```python
from build123d import *

# Parameters (mm, degrees)
SKETCH1_R             = 4.05
BOSS_EXTRUDE1_DEPTH   = 10
SKETCH2_W             = 18
SKETCH2_H             = 10
BOSS_EXTRUDE2_DEPTH   = 25
F_4_CLEARANCE_HOLE1_D = 3.2639


with BuildPart() as part:
    # Sketch1 → Boss-Extrude1 (new, symmetric)
    with BuildSketch(Plane.XY):
        with BuildLine():
            Line((-77.5, 0), (77.5, 0))
            Line((77.5, 0), (77.5, 7.5))
            ThreePointArc((77.5, 7.5), (75.303300859, 12.803300859), (70, 15))
            Line((70, 15), (60.5, 15))
            Line((60.5, 15), (60.5, 49.5))
            Line((60.5, 49.5), (42.5, 49.5))
            Line((42.5, 49.5), (42.5, 15))
            Line((42.5, 15), (-42.5, 15))
            Line((-42.5, 15), (-42.5, 49.5))
            Line((-42.5, 49.5), (-60.5, 49.5))
            Line((-60.5, 49.5), (-60.5, 15))
            Line((-60.5, 15), (-70, 15))
            ThreePointArc((-70, 15), (-75.303300859, 12.803300859), (-77.5, 7.5))
            Line((-77.5, 7.5), (-77.5, 0))
        make_face()
        with Locations((-70, 7.5)):
            Circle(SKETCH1_R, mode=Mode.SUBTRACT)
        with Locations((70, 7.5)):
            Circle(SKETCH1_R, mode=Mode.SUBTRACT)
    extrude(amount=BOSS_EXTRUDE1_DEPTH, both=True)

    # Sketch2 → Boss-Extrude2 (add)
    with BuildSketch(Plane(origin=(0, 49.5, 0), x_dir=(1, 0, 0), z_dir=(0, 1, 0))):
        with Locations((51.5, 5)):
            Rectangle(SKETCH2_W, SKETCH2_H)
        with Locations((-51.5, 5)):
            Rectangle(SKETCH2_W, SKETCH2_H)
    extrude(amount=BOSS_EXTRUDE2_DEPTH)

    # #4 Clearance Hole1 (through all)
    with Locations(Plane.XY):
        with Locations((-51.5, 64.5), (51.5, 64.5)):
            Hole(F_4_CLEARANCE_HOLE1_D / 2)


solid = part.part
```
Work out the finished part from the listing and answer in its coordinate system (mm). A direction names the side the tool comes from. Give positions to 0.01 mm unless a question says otherwise; leave off trailing zeros. Loops run counter-clockwise (first coordinate to the right, second up) from the corner with the lowest first, then second, coordinate; pieces in that order, holes last. Notation, with made-up numbers: (-6.5, 49.25) -> (44.5, 49.25) arc R23 ccw to (44.5, 71.25) -> close; hole circle Ø8 at (-12, -6). An arc over 180 degrees is marked (long way). Put each result on its own line as item: value. Start each with the question number.
Item 1: The mould has two halves that part along Y. Classify faces 1 (the face through (52, 49.5, 5)), 2 (the face through (-42.5, 38, -2)), 3 (the face through (51.854, 62.907, -5.07)), 4 (the face through (-66.26, 5.95, -0.14)): released by +Y, released by -Y, zero draft, split by the parting line, or undercut.
Item 2: Each of these flat-tipped pins is pushed along its axis until it touches: P1, Ø9, axis at x = 51.5, y = 62.5, coming from the +Z side; P2, Ø8, axis at x = -53.5, z = 5, coming from the +Y side; P3, Ø5, axis at x = -64.5, z = 1.5, coming from the +Y side; P4, Ø8, axis at y = 58, z = 7, coming from the -X side. Where does it stop, or does it pass through?
Item 3: Which of the six approach directions +Z, -Z, +X, -X, +Y, -Y give full straight-line access (tool end or side, diameter ignored) to faces 5 (the face through (-65, 15, 0)), 6 (the face through (-52, 62, 0)), 7 (the face through (65, 15, 0))?
Item 4: The part is cut by section C-C (z = -1.75). Give the vertices of the cut face in (x, y).
Item 5: The part is cut by section A-A (y = 64.5). Give the vertices of the cut face in (x, z).
Item 6: The part is cut by section D-D (y = 22.5). Give the vertices of the cut face in (x, z), then the cut area to 3 significant figures.
Item 7: Find the intervals of material crossed by L1, parallel to X at y = 7, z = 1.25; L2, parallel to X at y = 64.5, z = -4.5; L3, parallel to X at y = 36, z = -3, in increasing order. Write a range as [from, to].
Item 8: The part is cut by section B-B (x = -51.5). Give the vertices of the cut face in (y, z).
Answers below:
1. face 1: released by +Y
1. face 2: zero draft
1. face 3: undercut
1. face 4: undercut
2. P1: z = 0
2. P2: y = 49.5
2. P3: y = 15
2. P4: through
3. face 5: +Z, -Z, -X, +Y
3. face 6: +Z, +X, -X, +Y
3. face 7: +Z, -Z, +X, +Y
4. outline: (-77.5, 0) -> (77.5, 0) -> (77.5, 7.5) arc R7.5 ccw to (70, 15) -> (60.5, 15) -> (60.5, 74.5) -> (42.5, 74.5) -> (42.5, 15) -> (-42.5, 15) -> (-42.5, 74.5) -> (-60.5, 74.5) -> (-60.5, 15) -> (-70, 15) arc R7.5 ccw to (-77.5, 7.5) -> close; hole circle Ø8.1 at (-70, 7.5); hole circle Ø3.26 at (-51.5, 64.5); hole circle Ø3.26 at (51.5, 64.5); hole circle Ø8.1 at (70, 7.5)
5. outline: (-60.5, -10) -> (-53.13, -10) -> (-53.13, 0) -> (-60.5, 0) -> close; (-49.87, -10) -> (-42.5, -10) -> (-42.5, 0) -> (-49.87, 0) -> close; (42.5, -10) -> (49.87, -10) -> (49.87, 0) -> (42.5, 0) -> close; (53.13, -10) -> (60.5, -10) -> (60.5, 0) -> (53.13, 0) -> close
6. outline: (-60.5, -10) -> (-42.5, -10) -> (-42.5, 10) -> (-60.5, 10) -> close; (42.5, -10) -> (60.5, -10) -> (60.5, 10) -> (42.5, 10) -> close
6. area: 720 mm2
7. L1: [-77.5, -74.02], [-65.98, 65.98], [74.02, 77.5]
7. L2: [-60.5, -53.13], [-49.87, -42.5], [42.5, 49.87], [53.13, 60.5]
7. L3: [-60.5, -42.5], [42.5, 60.5]
8. outline: (0, -10) -> (62.87, -10) -> (62.87, 0) -> (49.5, 0) -> (49.5, 10) -> (0, 10) -> close; (66.13, -10) -> (74.5, -10) -> (74.5, 0) -> (66.13, 0) -> close
